Input: part model. Units: mm. Frame: model coordinates. Face numbers are marked on the shaded views. Give positions to 0.01 mm unless a question says otherwise; leave off trailing zeros. Loops run counter-clockwise (first coordinate to the right, second up) from the corner with the lowest first, then second, coordinate; pieces in that order, holes last. Notation, with made-up numbers: (-16, 85.5) -> (1, 85.5) arc R31 cw to (1, 114.5) -> close; hole circle Ø9 at (84.25, 16.5). An arc over 180 degrees is marked (long way). One line per question, with ' | ' between items.
from build123d import *

# Parameters (mm, degrees)
SKETCH1_R           = 2.1
SKETCH1_R_2         = 4
SKETCH1_R_3         = 8
BOSS_EXTRUDE1_DEPTH = 5
SKETCH2_R           = 15
CUT_EXTRUDE1_DEPTH  = 10


with BuildPart() as part:
    # Sketch1 → Boss-Extrude1 (new body)
    with BuildSketch(Plane.XY):
        Polygon((116.611470678, 15.338509317), (51.611470678, 15.338509317), (51.611470678, -6.661490683), (51.611470678, -24.661490683), (116.611470678, -24.661490683), (134.111470678, -24.661490683), (134.111470678, -6.661490683), align=None)
        with Locations((56.611470678, 10.338509317)):
            Circle(SKETCH1_R, mode=Mode.SUBTRACT)
        with Locations((111.611470678, 10.338509317)):
            Circle(SKETCH1_R, mode=Mode.SUBTRACT)
        with Locations((56.611470678, 0.338509317)):
            Circle(SKETCH1_R, mode=Mode.SUBTRACT)
        with Locations((111.611470678, 0.338509317)):
            Circle(SKETCH1_R, mode=Mode.SUBTRACT)
        with Locations((115.611470678, -12.661490683)):
            Circle(SKETCH1_R_2, mode=Mode.SUBTRACT)
        with Locations((90.611470678, -12.661490683)):
            Circle(SKETCH1_R_3, mode=Mode.SUBTRACT)
        with Locations((78.111470678, -12.661490683)):
            Circle(SKETCH1_R, mode=Mode.SUBTRACT)
        with Locations((103.111470678, -12.661490683)):
            Circle(SKETCH1_R, mode=Mode.SUBTRACT)
        with Locations((128.111470678, -12.661490683)):
            Circle(SKETCH1_R, mode=Mode.SUBTRACT)
    extrude(amount=BOSS_EXTRUDE1_DEPTH)

    # Sketch2 → Cut-Extrude1 (cut)
    with BuildSketch(Plane.XY.offset(5)):
        with Locations((90.611470678, 15.338509317)):
            Circle(SKETCH2_R)
    extrude(amount=-CUT_EXTRUDE1_DEPTH, mode=Mode.SUBTRACT)


solid = part.part
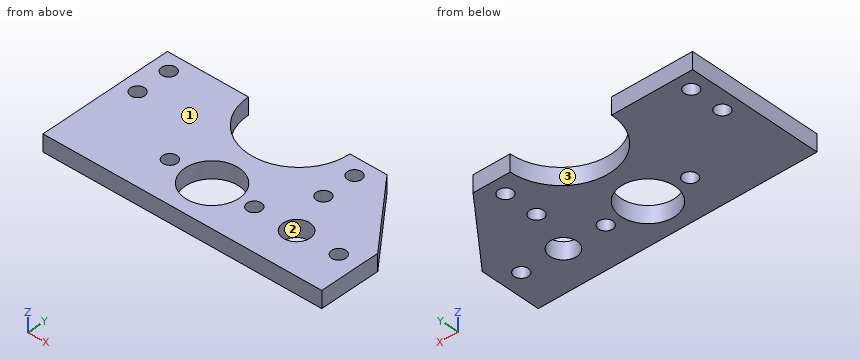
1. Ray query, line 1 along Y through (x, z) = (110.5, 4.5); line 2 along X through (y, z) = (-10.5, 0.95); line 3 along X through (y, z) = (-9.5, 1.25). Return the intervals inside material, ascending. Write a range as from..to.
Determined:
line 1: y = -24.66..-1.44, 2.12..8.56, 12.12..15.34 | line 2: x = 51.61..82.91, 98.31..112.25, 118.98..134.11 | line 3: x = 51.61..83.26, 97.96..113.16, 118.06..134.11
2. Section query D-D (z = 1.8). Count the separate pieces of the cut face and the enclosed holes in it, then the cut area to 3 significant figures.
Determined:
separate pieces: 1 | enclosed holes: 9 | area: 2,410 mm2
3. Pin query (flat end, axial travel): P1, Ø1.5, axis at x = 98, z = 3, coming from the +Y side. Return the tip coordinate at first contact, or that it passes through.
Determined:
P1: stops at y = 2.74
4. Section query B-B (y = 9). Output: boundary loops of the cut face in (x, z), then the cut area to 3 significant figures.
Determined:
outline: (51.61, 0) -> (54.99, 0) -> (54.99, 5) -> (51.61, 5) -> close; (58.23, 0) -> (77.02, 0) -> (77.02, 5) -> (58.23, 5) -> close; (104.21, 0) -> (109.99, 0) -> (109.99, 5) -> (104.21, 5) -> close; (113.23, 0) -> (121.65, 0) -> (121.65, 5) -> (113.23, 5) -> close | area: 182 mm2
5. Pull-direction query (Y, two-part tool) for the marked faces 1, 2 and 3; classes: pulls with the +Y half, pulls with the -Y half, needs draft (parallel to the pull), parting line crosses it, or undercut.
Determined:
face 1: needs draft | face 2: undercut | face 3: pulls with the +Y half
6. Section query C-C (y = -15.5). Output: boundary loops of the cut face in (x, z).
Determined:
outline: (51.61, 0) -> (83.13, 0) -> (83.13, 5) -> (51.61, 5) -> close; (98.09, 0) -> (112.79, 0) -> (112.79, 5) -> (98.09, 5) -> close; (118.43, 0) -> (134.11, 0) -> (134.11, 5) -> (118.43, 5) -> close
7. Section query A-A (x = 129). Output: boundary loops of the cut face in (y, z), then the cut area to 3 significant figures.
Determined:
outline: (-24.66, 0) -> (-14.56, 0) -> (-14.56, 5) -> (-24.66, 5) -> close; (-10.76, 0) -> (-0.24, 0) -> (-0.24, 5) -> (-10.76, 5) -> close | area: 103 mm2
